```python
from build123d import *

# Parameters (mm, degrees)
PAD_DEPTH       = 0.88
PAD_DEPTH_BACK  = 0.88
FILLET_R        = 2
SKETCH002_R     = 7.93
POCKET_DEPTH    = 5
POCKET001_DEPTH = 5


with BuildPart() as part:
    # Sketch → Pad (new body, two sides)
    with BuildSketch(Plane.XY) as pad_sk:
        with BuildLine():
            ThreePointArc((-0.875, 12.469337), (-12.5, 0), (-0.875, -12.469337))
            Line((-0.875, -12.469337), (-0.875, -16.469337))
            Line((-0.875, -16.469337), (0.875, -16.469337))
            Line((0.875, -12.469337), (0.875, -16.469337))
            ThreePointArc((0.875, -12.469337), (10.995688, -5.945153), (10.912848, 6.095879))
            Line((8.838835, 6.095879), (10.912848, 6.095879))
            ThreePointArc((6.698177, 10.553882), (6.366174, 7.651504), (8.838835, 6.095879))
            ThreePointArc((6.698177, 10.553882), (3.905828, 11.874111), (0.875, 12.469337))
            Line((0.875, 12.469337), (0.875, 16.469337))
            Line((-0.875, 16.469337), (0.875, 16.469337))
            Line((-0.875, 12.469337), (-0.875, 16.469337))
        make_face()
    extrude(amount=PAD_DEPTH)
    extrude(pad_sk.sketch, amount=-PAD_DEPTH_BACK)

    # Fillet
    fillet_edges = [part.edges().sort_by_distance(p)[0] for p in [
        (6.698177, 10.553882, 0),
        (10.912848, 6.095879, 0),
    ]]
    fillet(fillet_edges, radius=FILLET_R)

    # Sketch001 → Groove (revolve, cut)
    with BuildSketch(Plane.XY):
        with BuildLine():
            Line((-0.875, 12.469337), (-1.427669, 12.469337))
            Line((-1.427669, 12.469337), (-1.427669, 16.923711))
            Line((-1.427669, 16.923711), (0, 16.923711))
            Line((0, 16.923711), (0, 16.469337))
            ThreePointArc((0, 16.469337), (-0.296631, 16.319125), (-0.4408, 16.01951))
            Line((-0.875, 12.469337), (-0.4408, 16.01951))
        make_face()
    groove = revolve(axis=Axis((0, 0, 0), (0, 1, 0)), mode=Mode.SUBTRACT)

    # Mirrored: Groove across XZ
    add(groove.mirror(Plane.XZ), mode=Mode.SUBTRACT)

    # Sketch002 (on Face6 of Mirrored) → Pocket (cut)
    with BuildSketch(Plane.XY.offset(0.88)):
        Circle(SKETCH002_R)
    extrude(amount=-POCKET_DEPTH, mode=Mode.SUBTRACT)

    # Sketch003 (on Face6 of Pocket) → Pocket001 (cut)
    with BuildSketch(Plane.XY.offset(0.88)):
        Polygon((12.882158, 5), (12.882158, -5), (11.456439, -5), (11.452158, 5), align=None)
    pocket001 = extrude(amount=-POCKET001_DEPTH, mode=Mode.SUBTRACT)

    # Mirrored001: Pocket001 across Sketch003 V_Axis
    add(pocket001.mirror(Plane(origin=(0, 0, 0.88), x_dir=(0, 0, 1), z_dir=(1, 0, 0))), mode=Mode.SUBTRACT)


solid = part.part
```
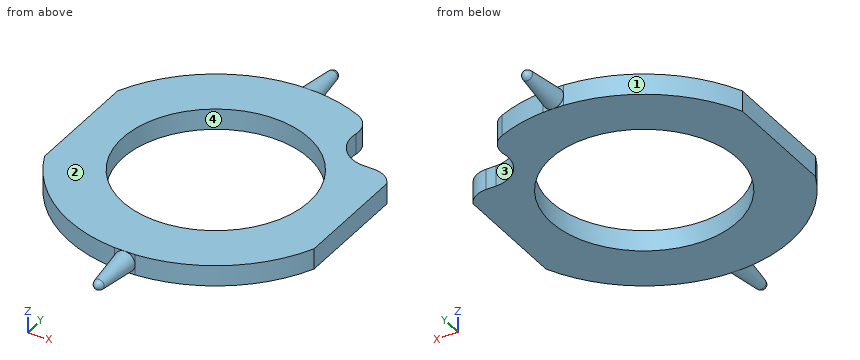
Here's how the part is built. I have some questions about the finished solid (model axes, mm). Face numbers are marked on the shaded views. Give positions to 0.01 mm unless a question says otherwise; leave off trailing zeros. Write each loop counter-clockwise with the first axis right and the second up, starting at its lowest first coordinate (ties: lowest second). Pieces come first, ordered by that corner, then holes. Notation, with made-up numbers: (12.25, -6) -> (62.25, -6) arc R20 cw to (62.25, 27) -> close; hole circle Ø3 at (43.5, 27). An arc over 180 degrees is marked (long way). Use one line per item in the form item = value.
1) We'd pull the mould along Y, two halves only. Please class the marked faces 1, 2, 3 and 4: +Y half, -Y half, draft (parallel to the pull), parting line (faces both ways), or undercut.
Verdict:
face_1 = +Y half
face_2 = draft
face_3 = undercut
face_4 = undercut
2) Suppose I cut it at C-C (y = -14). Please give me the cut outline in (x, z).
Verdict:
outline = circle Ø1.38 at (0, 0)
3) I'm going to push flat-ended pins straight in: pin 1 (0.7 mm diameter, centred on x = 0, z = -0.5, fed in from +Y); pin 2 (0.9 mm diameter, centred on y = 1, z = -0.5, fed in from +X); pin 3 (12.5 mm diameter, centred on x = 0, y = 0, fed in from +Z); pin 4 (0.7 mm diameter, centred on x = 0, z = 0.5, fed in from -Y). Where does each tip first touch, or does it pass through?
Verdict:
pin_1 = 16.42
pin_2 = 11.45
pin_3 = through
pin_4 = -16.42
4) Suppose I cut it at A-A (x = -4.25). Please give me the cut outline in (y, z), and give its area (3 significant figures).
Verdict:
outline = (-11.76, -0.88) -> (-6.69, -0.88) -> (-6.69, 0.88) -> (-11.76, 0.88) -> close; (6.69, -0.88) -> (11.76, -0.88) -> (11.76, 0.88) -> (6.69, 0.88) -> close
area = 17.8 mm2
5) Suppose I cut it at B-B (y = -7). Please give me the cut outline in (x, z), and give its area (3 significant figures).
Verdict:
outline = (-10.36, -0.88) -> (-3.73, -0.88) -> (-3.73, 0.88) -> (-10.36, 0.88) -> close; (3.73, -0.88) -> (10.36, -0.88) -> (10.36, 0.88) -> (3.73, 0.88) -> close
area = 23.3 mm2
6) If I drill on L1, parallel to Y at x = -6.75, z = 0.05; L2, parallel to X at y = 3.5, z = 0; L3, parallel to Y at x = -1, z = -0.8, over which ranges is the centre line in solid material (lowest first)? Write a range as [from, to].
Verdict:
L1 = [-10.52, -4.16], [4.16, 10.52]
L2 = [-11.45, -7.12], [7.12, 11.45]
L3 = [-12.46, -7.87], [7.87, 12.46]
